from build123d import *

# Parameters (mm, degrees)
F0_W         = 762
F0_H         = 1438.275
F1_DEPTH     = 3.175
F2_W         = 762
F2_H         = 1438.275
F2_W_2       = 755.65
F2_H_2       = 1431.925
F3_DEPTH     = 28.575
F4_R         = 5.08
F5_T1_DEPTH  = 39.37
F5_S5_W      = 5.1816
F5_S5_H      = 5.1816
F5_T6_DEPTH  = 5.1816
F5_S11_W     = 5.1816
F5_S11_H     = 5.1816
F5_T12_DEPTH = 5.1816
F5_S17_W     = 5.1816
F5_S17_H     = 5.1816
F5_T18_DEPTH = 5.1816
F5_S23_W     = 5.1816
F5_S23_H     = 5.1816
F5_T24_DEPTH = 5.1816


# Not quite as in the source:
# - a fillet or chamfer that OpenCascade refuses, or shapes differently, is made with other operations: its cross-section is extruded or revolved along the edge and cut away or added


with BuildPart() as f1:
    # F0 (on Front) → F1 (new body)
    with BuildSketch(Plane.XZ):
        Rectangle(F0_W, F0_H)
    extrude(amount=F1_DEPTH)

    # F2 (on face) → F3 (join)
    with BuildSketch(Plane.XZ.offset(3.175)):
        Rectangle(F2_W, F2_H)
        Rectangle(F2_W_2, F2_H_2, mode=Mode.SUBTRACT)
    extrude(amount=F3_DEPTH)

    # F4
    f4_edges = [f1.edges().sort_by_distance(p)[0] for p in [
        (0, 0, -719.1375),
        (381, 0, 0),
        (-381, 0, 0),
        (0, 0, 719.1375),
    ]]
    fillet(f4_edges, radius=F4_R)

    # F5: fillet of radius 5.08 on 4 edges, made by hand

    # F5_s2 → F5_t1 (cut)
    with BuildSketch(Plane.XZ.offset(5.08)):
        with BuildLine():
            ThreePointArc((-381, 714.0575), (-379.5121024484, 717.6496024484), (-375.92, 719.1375))
            Line((-375.92, 719.1375), (-381, 719.1375))
            Line((-381, 719.1375), (-381, 714.0575))
        make_face()
        with BuildLine():
            ThreePointArc((375.92, 719.1375), (379.5121024484, 717.6496024484), (381, 714.0575))
            Line((381, 714.0575), (381, 719.1375))
            Line((381, 719.1375), (375.92, 719.1375))
        make_face()
        with BuildLine():
            ThreePointArc((375.92, -719.1375), (379.5121024484, -717.6496024484), (381, -714.0575))
            Line((381, -714.0575), (381, -719.1375))
            Line((381, -719.1375), (375.92, -719.1375))
        make_face()
        with BuildLine():
            ThreePointArc((-381, -714.0575), (-379.5121024484, -717.6496024484), (-375.92, -719.1375))
            Line((-375.92, -719.1375), (-381, -719.1375))
            Line((-381, -719.1375), (-381, -714.0575))
        make_face()
    extrude(amount=F5_T1_DEPTH, mode=Mode.SUBTRACT)


with BuildPart() as f5_tool4:
    # F5_s5 → F5_t6 (new body)
    with BuildSketch(Plane.YZ.offset(-375.92)):
        with Locations((-2.4892, -716.6483)):
            Rectangle(F5_S5_W, F5_S5_H)
    extrude(amount=-F5_T6_DEPTH)

    # F5_s7 → F5_t8 (revolve, cut)
    with BuildSketch(Plane(origin=(-375.92, -5.08, -714.0575), x_dir=(0, -0.7071067812, 0.7071067812), z_dir=(0, -0.7071067812, -0.7071067812))):
        with BuildLine():
            ThreePointArc((0, -5.08), (5.08, 0), (0, 5.08))
            Line((0, 5.08), (0, -5.08))
        make_face()
    revolve(axis=Axis((-375.92, -5.08, -714.0575), (-1, 0, 0)), mode=Mode.SUBTRACT)


with BuildPart() as f1_1:
    add(f1.part)

    # F5_t3: cut F5_tool4
    add(f5_tool4.part, mode=Mode.SUBTRACT)


with BuildPart() as f5_tool10:
    # F5_s11 → F5_t12 (new body)
    with BuildSketch(Plane.XY.offset(-714.0575)):
        with Locations((378.5108, -2.4892)):
            Rectangle(F5_S11_W, F5_S11_H)
    extrude(amount=-F5_T12_DEPTH)

    # F5_s13 → F5_t14 (revolve, cut)
    with BuildSketch(Plane(origin=(375.92, -5.08, -714.0575), x_dir=(-0.7071067812, -0.7071067812, 0), z_dir=(0.7071067812, -0.7071067812, 0))):
        with BuildLine():
            ThreePointArc((0, -5.08), (5.08, 0), (0, 5.08))
            Line((0, 5.08), (0, -5.08))
        make_face()
    revolve(axis=Axis((375.92, -5.08, -714.0575), (0, 0, -1)), mode=Mode.SUBTRACT)


with BuildPart() as f1_2:
    add(f1_1.part)

    # F5_t9: cut F5_tool10
    add(f5_tool10.part, mode=Mode.SUBTRACT)


with BuildPart() as f5_tool16:
    # F5_s17 → F5_t18 (new body)
    with BuildSketch(Plane.XY.offset(714.0575)):
        with Locations((378.5108, -2.4892)):
            Rectangle(F5_S17_W, F5_S17_H)
    extrude(amount=F5_T18_DEPTH)

    # F5_s19 → F5_t20 (revolve, cut)
    with BuildSketch(Plane(origin=(375.92, -5.08, 714.0575), x_dir=(-0.7071067812, -0.7071067812, 0), z_dir=(-0.7071067812, 0.7071067812, 0))):
        with BuildLine():
            ThreePointArc((0, -5.08), (5.08, 0), (0, 5.08))
            Line((0, 5.08), (0, -5.08))
        make_face()
    revolve(axis=Axis((375.92, -5.08, 714.0575), (0, 0, 1)), mode=Mode.SUBTRACT)


with BuildPart() as f1_3:
    add(f1_2.part)

    # F5_t15: cut F5_tool16
    add(f5_tool16.part, mode=Mode.SUBTRACT)


with BuildPart() as f5_tool22:
    # F5_s23 → F5_t24 (new body)
    with BuildSketch(Plane.YZ.offset(-375.92)):
        with Locations((-2.4892, 716.6483)):
            Rectangle(F5_S23_W, F5_S23_H)
    extrude(amount=-F5_T24_DEPTH)

    # F5_s25 → F5_t26 (revolve, cut)
    with BuildSketch(Plane(origin=(-375.92, -5.08, 714.0575), x_dir=(0, -0.7071067812, -0.7071067812), z_dir=(0, 0.7071067812, -0.7071067812))):
        with BuildLine():
            ThreePointArc((0, -5.08), (5.08, 0), (0, 5.08))
            Line((0, 5.08), (0, -5.08))
        make_face()
    revolve(axis=Axis((-375.92, -5.08, 714.0575), (-1, 0, 0)), mode=Mode.SUBTRACT)


with BuildPart() as f1_4:
    add(f1_3.part)

    # F5_t21: cut F5_tool22
    add(f5_tool22.part, mode=Mode.SUBTRACT)


solid = f1_4.part
Can you work these out from the model? Positions are in its coordinate system, mm. A direction names the side the tool comes from. Coordinates: 2 decimals unless noted, no trailing zeros. Order: outer loops, then holes, each group sorted by start corner. A loop starts at its lowest first (then second) coordinate and runs counter-clockwise, first axis right, second up. Notation, with made-up numbers: (45.5, 72) - (68.5, 72) arc R20 cw to (68.5, 82) - close; hole circle Ø5 at (-1, -35). An arc over 180 degrees is marked (long way). Answer as a JSON object with one key per item and string values. Group by question number.
Q1. Imagine slicing it at A-A (y = -15). Please give me the cut outline in (x, z) (1 decimal), and give its area (3 significant figures).
Q2. Imagine slicing it at B-B (z = 294). Please give me the cut outline in (x, y) (3 decimals), and give its area (3 significant figures).
Q3. We'd pull the mould along Z, two halves only. Please class faces 1 (the face through (377.825, -17, -10)), 2 (the face through (-5, -18, 719.138)), 3 (the face through (-381, -18, -10)): +Z half, -Z half, draft (parallel to the pull), parting line (faces both ways), or undercut.
Q4. On a 3-axis mill with a long thin cutter (end or side, diameter ignored), from which of +Z, -Z, +X, -X, +Y, -Y can I reach the whole of each face in a straight line? I mean faces 4 (the face through (-5, -3.175, 10)), 5 (the face through (-5, 0, 10)). Say none if no direction works.
Q5. I need wall thicknesses on line 1 (X direction, y = -22.5, z = -611) (3 decimals); line 2 (Z direction, x = -116, y = -9.5); line 3 (Z direction, x = 180, y = -4). Which ranges of each line are inside material? Lowest first, please. Write a range as from..to.
Q6. Will this pin go through, and if not, where does the flat tip stop? P1, Ø10, axis at x = 89.5, z = 451.5, coming from the -Y side (3 decimals).
Determined:
{
 "1": {"outline": "(-381, -714.1) arc R5.1 ccw to (-375.9, -719.1) - (375.9, -719.1) arc R5.1 ccw to (381, -714.1) - (381, 714.1) arc R5.1 ccw to (375.9, 719.1) - (-375.9, 719.1) arc R5.1 ccw to (-381, 714.1) - close; hole (-377.8, -716) - (377.8, -716) - (377.8, 716) - (-377.8, 716) - close", "area": "13,900 mm2"},
 "2": {"outline": "(-381, -31.75) - (-377.825, -31.75) - (-377.825, -3.175) - (377.825, -3.175) - (377.825, -31.75) - (381, -31.75) - (381, -5.08) arc R5.08 ccw to (375.92, 0) - (-375.92, 0) arc R5.08 ccw to (-381, -5.08) - close", "area": "2,590 mm2"},
 "3": {"face 1": "undercut", "face 2": "+Z half", "face 3": "draft"},
 "4": {"face 4": "-Y", "face 5": "+Z, -Z, +X, -X, +Y"},
 "5": {"line 1": "x = -381..-377.825, 377.825..381", "line 2": "z = -719.14..-715.96, 715.96..719.14", "line 3": "z = -719.02..-715.96, 715.96..719.02"},
 "6": {"P1": "stops at y = -3.175"}
}
